Geometry check sheet. Reference: the model listing, model coordinates, mm. A direction names the side the tool comes from. Round coordinates to 2 decimals unless told otherwise and drop trailing zeros. Loops run counter-clockwise (first coordinate to the right, second up) from the corner with the lowest first, then second, coordinate; pieces in that order, holes last. Notation, with made-up numbers: (43, -10) -> (59, -10) arc R22 cw to (59, 26) -> close; hole circle Ø8 at (82.5, -2.75). An arc over 180 degrees is marked (long way). Use a Markdown table: item, result. Add a question column.
Q1. Material ranges on L1, parallel to Y at x = -37.15, z = -35.3; L2, parallel to Y at x = -28, z = -18.5; L3, parallel to Z at x = -35, y = 3, recorded low to high.
Q2. Sectioned sample at C-C, the plane x = -7. Enter the section's corners in (y, z).
Q3. Sectioned sample at B-B, the plane z = -10.3. Enter the section's corners in (x, y).
Q4. Sectioned sample at D-D, the plane x = -17.5. Enter the section's corners in (y, z), then the cut area to 3 significant figures.
Q5. Gauge pin test, flat ends, axial feed: P1, Ø3, axis at x = -5.5, y = 3.5, coming from the -Z side; P2, Ø4.5, axis at y = -1.5, z = -36.5, coming from the -X side; P3, Ø2.5, axis at x = -11.5, y = -1, coming from the +Z side; P4, Ø1.2, axis at x = -35, z = -27.1, coming from the +Y side. Record the tip position at first contact, or that the pin passes through.
Q6. Set-up check for faces 1 (the face through (-11, -1, -32.3)), 2 (the face through (-37.6, 0.9, 5.1)), 3 (the face through (-39.5, 4, -33)), 4 (the face through (-5.551, 4.684, 2.387)), 5 (the face through (-35.8, -4, -36)): record each of +Z, -Z, +X, -X, +Y, -Y from which the full face is reachable in a straight line by a thin tool's end or side.
Q7. Release check for a two-part mould opening along Z. For faces 6 (the face through (-5, 5, -30)), 7 (the face through (-37.68, -5.38, -35.37)), 8 (the face through (-37.68, -3.29, -36.49)) record: released by +Z, released by -Z, zero draft, split by the parting line, or undercut.
Q8. Sectioned sample at A-A, the plane z = -35.3. Enter the section's corners in (x, y).
Autodesk Inventor part; units mm, degrees
ref_plane "YZ Plane" through (0, 0, 0) normal (1, 0, 0) x (0, 1, 0)
ref_plane "XZ Plane" through (0, 0, 0) normal (0, 1, 0) x (-1, 0, 0)
ref_plane "XY Plane" through (0, 0, 0) normal (0, 0, 1) x (1, 0, 0)
sketch "Skizze1" plane through (0, 0, 0) normal (0, 1, 0) x (-1, 0, 0)
  line L0 (0, 0) -> (0, -30)
  line L1 (0, -30) -> (9.5, -30)
  line L2 (9.5, -30) -> (9.5, -38.3)
  line L3 (9.5, -38.3) -> (39.5, -38.3)
  line L4 (39.5, -38.3) -> (39.5, -28)
  line L5 (39.5, -28) -> (42.7, -28)
  line L6 (42.7, -28) -> (42.7, -23.4)
  arc A0 (37.6, 2.1) -> (42.7, -23.4) centre (45.7856, -9.5229) ccw
  line L7 (0, 0) -> (11.2599, 4.8422)
  line L8 (11.2599, 4.8422) -> (4.7414, 20)
  line L9 (4.7414, 20) -> (24.5844, 28.5332)
  line L10 (24.5844, 28.5332) -> (33.3715, 8.1)
  line L11 (62.1927, -61.79) -> (-17.9865, -61.79) construction
  line L12 (-17.9865, -61.79) -> (-17.9865, 45.1157) construction
  line L13 (-17.9865, 45.1157) -> (62.1927, 45.1157) construction
  line L14 (62.1927, 45.1157) -> (62.1927, -61.79) construction
  line L15 (-1.7899, 2.1) -> (7.9361, 5.9872)
  line L16 (37.6, 2.1) -> (37.6, 8.1)
  line L17 (37.6, 8.1) -> (33.3715, 8.1)
  dimension "d0" = 30
  dimension "d1" = 9.5
  dimension "d2" = 8.3
  dimension "d3" = 30
  dimension "d4" = 10.3
  dimension "d5" = 3.2
  dimension "d6" = 4.6
  dimension "d7" = 5.1
  dimension "d8" = 25.5
  dimension "d10" = 90
  dimension "d11" = 20
  dimension "d12" = 16.5
  dimension "d13" = 21.6
  dimension "d14" = 90
  dimension "d30" = 90
  dimension "d34" = 6
extrude "Extrusion1" add sketch "Skizze1" along normal blind 9.5
sketch "Skizze2" plane through (-24.5844, 0, 28.5332) normal (-0.9187, 0, 0.3951) x (0.3951, 0, 0.9187)
  line L0 (-22.2425, 0) -> (0, 0)
  line L1 (0, 0) -> (0, 9.5)
  line L2 (-22.2425, 9.5) -> (0, 9.5)
  line L3 (-22.2425, 0) -> (-22.2425, 9.5)
  circle A0 centre (-14.3, 4.75) radius 1.5
  point P0 (-16.5, 0)
  dimension "d38" = 14.3
  dimension "d39" = 3
extrude "Extrusion2" cut sketch "Skizze2" against normal blind 9.5 contours A0
sketch "Skizze3" plane through (-39.5, 0, -38.3) normal (-1, 0, 0) x (0, 0, 1)
  line L0 (0, 0) -> (10.3, 0)
  line L1 (10.3, 0) -> (10.3, 9.5)
  line L2 (0, 9.5) -> (10.3, 9.5)
  line L3 (0, 0) -> (0, 9.5)
  circle A0 centre (3, -2.3798) radius 1.5
  circle A1 centre (3, -2.3798) radius 3
  line L4 (0, 0) -> (0, 9.5)
  line L5 (0, -2.3798) -> (0, 0.1566)
  line L6 (6, -2.3798) -> (6, 0)
  line L7 (8.3, 0) -> (0, 0)
  point P0 (38.3, 0)
  dimension "d42" = 3
  dimension "d43" = 6
extrude "Extrusion3" add sketch "Skizze3" against normal up to surface (30 mm away) contours L6 A1 L0 | A1 L0 | A1 L5 L0 picked at (2.9397, -0.2969)
sketch "Skizze4" plane through (0, 0, 0) normal (0, -1, 0) x (1, 0, 0)
  line L0 (-39.5, -32.3) -> (-9.5, -32.3)
  line L1 (-9.5, -30) -> (-9.5, -32.3)
  line L2 (0, -30) -> (-9.5, -30)
  line L3 (0, 0) -> (0, -30)
  line L4 (-11.2599, 4.8422) -> (0, 0)
  line L5 (-4.7414, 20) -> (-11.2599, 4.8422)
  line L6 (-24.5844, 28.5332) -> (-4.7414, 20)
  line L7 (-33.3715, 8.1) -> (-24.5844, 28.5332)
  line L8 (-37.6, 8.1) -> (-33.3715, 8.1)
  line L9 (-37.6, 2.1) -> (-37.6, 8.1)
  arc A0 (-42.7, -23.4) -> (-37.6, 2.1) centre (-45.7856, -9.5229) ccw
  line L10 (-42.7, -28) -> (-42.7, -23.4)
  line L11 (-39.5, -28) -> (-42.7, -28)
  line L12 (-39.5, -32.3) -> (-39.5, -28)
  circle A1 centre (-25, -10.3) radius 3.4826
  line L13 (-39.5, -38.3) -> (-9.5, -38.3)
  dimension "d46" = 25
  dimension "d47" = 28
extrude "Extrusion4" cut sketch "Skizze4" against normal blind 10 contours A1
sketch "Skizze5" plane through (0, 0, 0) normal (0, -1, 0) x (1, 0, 0)
  line L0 (-9.5, -38.3) -> (-9.5, -32.3)
  line L1 (-39.5, -32.3) -> (-9.5, -32.3)
  line L2 (-39.5, -38.3) -> (-39.5, -32.3)
  line L3 (-39.5, -38.3) -> (-9.5, -38.3)
  line L4 (-9.5, -38.3) -> (-39.5, -38.3)
  line L5 (-35.8, -32.3) -> (-13.24, -32.3)
  line L6 (-13.24, -32.3) -> (-13.24, -38.3)
  line L7 (-13.24, -38.3) -> (-35.8, -38.3)
  line L8 (-35.8, -38.3) -> (-35.8, -32.3)
  line L9 (-13.24, -32.3) -> (-35.8, -32.3)
  line L10 (-35.8, -32.3) -> (-35.8, -38.3)
  line L11 (-35.8, -38.3) -> (-13.24, -38.3)
  line L12 (-13.24, -38.3) -> (-13.24, -32.3)
  point P0 (0, 0)
  dimension "d50" = 3.74
  dimension "d51" = 3.7
extrude "Extrusion5" cut sketch "Skizze5" along normal blind 10 contours L3 L8 L1 L6
sketch "Skizze6" plane through (0, 0, 0) normal (0, -1, 0) x (1, 0, 0)
  arc A0 (-36.7, -25.4555) -> (-37.7, -26.4555) centre (-36.7, -26.4555) ccw
  line L0 (-37.7, -26.4555) -> (-37.7, -29.6)
  line L1 (-37.7, -29.6) -> (-12, -29.6)
  line L2 (-12, -29.6) -> (-12, -20.0723)
  arc A1 (-12, -20.0723) -> (-13, -19.0723) centre (-13, -20.0723) ccw
  line L3 (-13, -19.0723) -> (-14.8624, -19.0723)
  arc A2 (-15.8624, -18.0723) -> (-14.8624, -19.0723) centre (-14.8624, -18.0723) ccw
  line L4 (-15.8624, -18.0723) -> (-15.8624, 0.4)
  line L5 (-15.8624, 0.4) -> (-27.397, 0.4)
  arc A3 (-28.397, 1.4) -> (-27.397, 0.4) centre (-27.397, 1.4) ccw
  line L6 (-28.397, 1.4) -> (-28.397, 2.4)
  arc A4 (-28.397, 2.4) -> (-29.397, 3.4) centre (-29.397, 2.4) ccw
  line L7 (-29.397, 3.4) -> (-31.9624, 3.4)
  arc A5 (-31.9624, 3.4) -> (-32.9624, 2.4) centre (-31.9624, 2.4) ccw
  line L8 (-32.9624, 2.4) -> (-32.9624, -24.4555)
  arc A6 (-33.9624, -25.4555) -> (-32.9624, -24.4555) centre (-33.9624, -24.4555) ccw
  line L9 (-33.9624, -25.4555) -> (-36.7, -25.4555)
  line L10 (-31, -17.1) -> (-31, -1.6)
  line L11 (-31, -1.6) -> (-17.5, -1.6)
  line L12 (-17.5, -1.6) -> (-17.5, -17.1)
  line L13 (-17.5, -17.1) -> (-31, -17.1)
  circle A7 centre (-35, -27.1) radius 1
  circle A8 centre (-14.5, -20.6) radius 1
  circle A9 centre (-30, 0.9) radius 1
  line L14 (-42.7, -28) -> (-42.7, -23.4)
  point P0 (0, 0)
  dimension "d56" = 7.7
extrude "Extrusion6" cut sketch "Skizze6" against normal through all contours A7 | A8 | A9
sketch "Skizze7" plane through (-24.5844, 0, 28.5332) normal (-0.9187, 0, 0.3951) x (0.3951, 0, 0.9187)
  circle A0 centre (-14.3, 4.75) radius 1.5
  line L0 (-22.2425, 0) -> (0, 0)
  line L1 (0, 0) -> (0, 9.5)
  line L2 (-22.2425, 9.5) -> (0, 9.5)
  line L3 (-22.2425, 0) -> (-22.2425, 9.5)
  line L4 (-29.4249, 0) -> (-23.913, 0)
  line L5 (-23.913, 0) -> (-23.913, 9.5)
  line L6 (-29.4249, 9.5) -> (-23.913, 9.5)
  line L7 (-29.4249, 0) -> (-29.4249, 9.5)
  line L8 (-23.913, 0) -> (-23.913, 9.5)
  line L9 (-23.913, 0) -> (-22.2425, 0)
  line L10 (-22.2425, 0) -> (-22.2425, 9.5)
  line L11 (-23.913, 9.5) -> (-22.2425, 9.5)
  line L12 (-23.913, 0) -> (-23.913, 9.5)
  line L13 (-22.2425, 0) -> (-22.2425, 9.5)
  line L14 (-29.4249, 0) -> (-29.4249, 9.5)
  line L15 (-22.2425, 1.1485) -> (-29.4249, 1.1485)
  line L16 (-29.4249, 1.1485) -> (-29.4249, 8.8348)
  line L17 (-29.4249, 8.8348) -> (-22.2425, 8.8348)
  line L18 (-22.2425, 8.8348) -> (-22.2425, 1.1485)
  point P0 (-16.5, 0)
  point P1 (-23.913, 8.8348)
  point P2 (-29.4249, 8.8348)
  point P3 (-23.913, 1.1485)
  point P4 (-23.913, 0)
  point P5 (-23.913, 9.5)
extrude "Extrusion7" cut sketch "Skizze7" along normal blind 10 contours L9 L5 L15 L3 | L15 L5 L17 L3 | L17 L5 L11 L3 | L15 L7 L17 L5
sketch "Skizze8" plane through (-24.5844, 0, 28.5332) normal (-0.9187, 0, 0.3951) x (0.3951, 0, 0.9187)
  line L0 (-16.5, 0) -> (-16.5, 9.5)
  circle A0 centre (-14.3, 4.75) radius 1.5
  line L1 (0, 0) -> (-23.913, 0)
  line L2 (0, 0) -> (0, 9.5)
  line L3 (-23.913, 9.5) -> (0, 9.5)
  line L4 (-23.913, 9.5) -> (-23.913, 8.8348)
  line L5 (-23.913, 8.8348) -> (-29.4249, 8.8348)
  line L6 (-29.4249, 8.8348) -> (-29.4249, 1.1485)
  line L7 (-29.4249, 1.1485) -> (-23.913, 1.1485)
  line L8 (-23.913, 1.1485) -> (-23.913, 0)
  circle A1 centre (-24.3, 4.75) radius 1
  dimension "d59" = 2
  dimension "d60" = 10
extrude "Extrusion8" cut sketch "Skizze8" against normal blind 10 contours A1
properties part number "00_KES400A_base"
Values:
| question | item | result |
|---|---|---|
| 1 | L1 | -5.38 to -3.88, -0.88 to 9.5 |
| 1 | L2 | 0 to 9.5 |
| 1 | L3 | -38.3 to -28.1, -26.1 to -18.78, -0.26 to 4.31 |
| 2 | outline | (0, -30) -> (9.5, -30) -> (9.5, 3.01) -> (0, 3.01) -> close; (0, 14.75) -> (9.5, 14.75) -> (9.5, 20.97) -> (0, 20.97) -> close |
| 3 | outline | (-31.59, 0) -> (-28.48, 0) -> (-28.48, 9.5) -> (-31.59, 9.5) -> close; (-21.52, 0) -> (0, 0) -> (0, 9.5) -> (-21.52, 9.5) -> close |
| 4 | outline | (0, -38.3) -> (9.5, -38.3) -> (9.5, 25.49) -> (0, 25.49) -> close |
| 4 | area | 606 mm^2 |
| 5 | P1 | z = -30 |
| 5 | P2 | x = -39.5 |
| 5 | P3 | z = 23.23 |
| 5 | P4 | through |
| 6 | face 1 | +Z, +X, -X, -Y |
| 6 | face 2 | +Z, -X, +Y, -Y |
| 6 | face 3 | -Z, -X, +Y, -Y |
| 6 | face 4 | +X, +Y, -Y |
| 6 | face 5 | +Z, -Z, -Y |
| 7 | face 6 | released by -Z |
| 7 | face 7 | split by the parting line |
| 7 | face 8 | undercut |
| 8 | outline | (-39.5, -5.38) -> (-35.8, -5.38) -> (-35.8, -3.88) -> (-39.5, -3.88) -> close; (-39.5, -0.88) -> (-35.8, -0.88) -> (-35.8, 0) -> (-13.24, 0) -> (-13.24, -0.88) -> (-9.5, -0.88) -> (-9.5, 9.5) -> (-39.5, 9.5) -> close; (-13.24, -5.38) -> (-9.5, -5.38) -> (-9.5, -3.88) -> (-13.24, -3.88) -> close |
